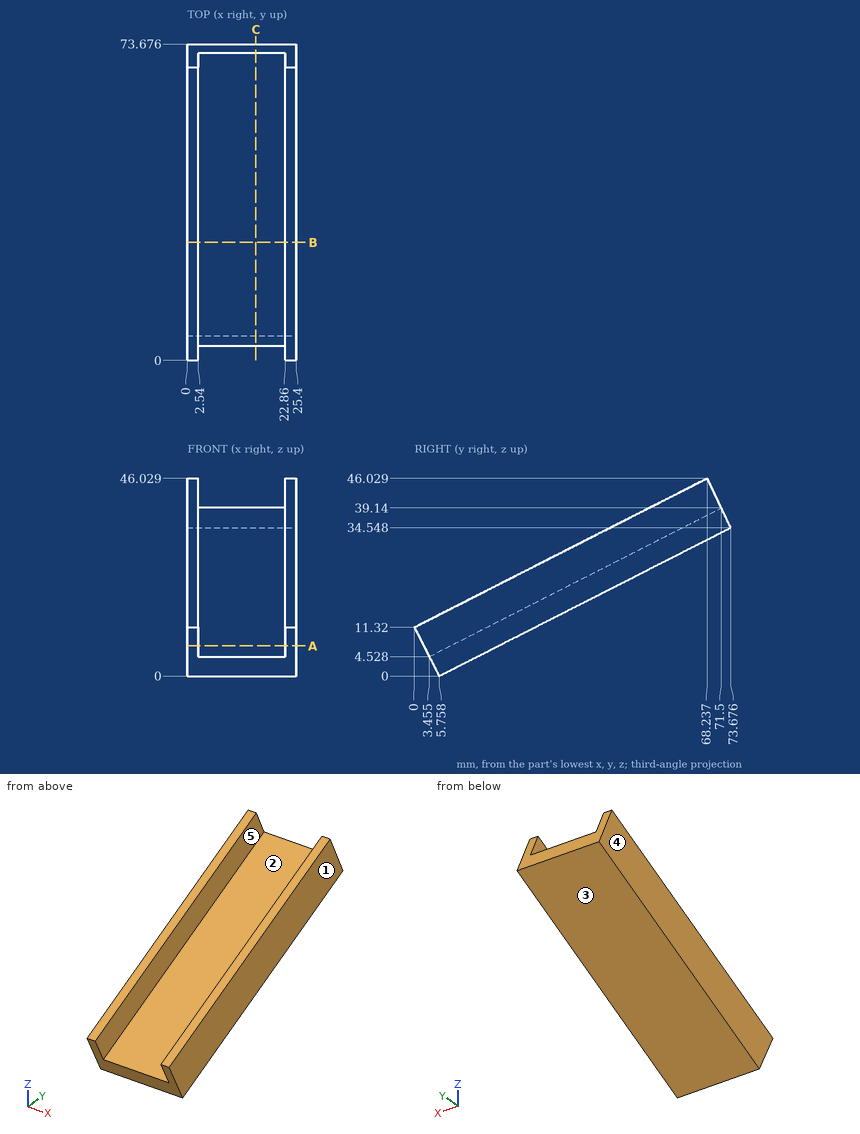
Study the drawing (mm; zero at the part's minimum x, y, z) and answer. A direction names the side the tool comes from. Round coordinates to 2 decimals unless told otherwise and drop trailing zeros. Write each loop counter-clockwise with the first axis right and the second up, starting at its lowest first coordinate (ties: lowest second). Pieces come first, ordered by that corner, then holes.
1) A cutting plane is placed at B-B (y = 27.5). Give the vertices of the cut face in (x, z), plus the area to 3 significant figures.
2) A cutting plane is placed at C-C (x = 16). Give the vertices of the cut face in (y, z) (1 decimal).
3) A cutting plane is placed at A-A (z = 7). Give the vertices of the cut face in (x, y) (1 decimal), plus the area to 3 significant figures.
4) Straight lines are drawn through the part: line 1 (Y direction, x = 2.75, z = 22) (1 decimal); line 2 (Y direction, x = 6, z = 2) (1 decimal); line 3 (Z direction, x = 3.5, y = 58) (1 decimal). For each, find the intervals that lie inside material, in ascending order.
5) Given pin 1 Ø1 at (x, z) = (11, 38) entering from -Y (1 decimal); pin 2 Ø10 at (x, z) = (14, 35) entering from -Y; pin 3 Ø8 at (x, y) = (17.5, 53) entering from +Z (1 decimal), each flat-ended and moving along its own axis, determine where each tip first touches the part or whether it passes through.
6) A tool of negligible diameter and unlimited length cuts with its end or side. For the marked faces 1 and 2, from which of +Z, -Z, +X, -X, +Y, -Y can it reach the whole face along a straight path? Write none if from no direction.
7) The mould has two halves that part along X. Classify the marked faces 3, 4 and 5: pulls with the +X half, pulls with the -X half, needs draft (parallel to the pull), parting line crosses it, or undercut.
Completed:
1. outline: (0, 11.06) - (25.4, 11.06) - (25.4, 25.31) - (22.86, 25.31) - (22.86, 16.76) - (2.54, 16.76) - (2.54, 25.31) - (0, 25.31) - close
1. area: 188 mm2
2. outline: (3.5, 4.5) - (5.8, 0) - (73.7, 34.5) - (71.5, 39.1) - close
3. outline: (0, 2.2) - (2.5, 2.2) - (2.5, 8.3) - (22.9, 8.3) - (22.9, 2.2) - (25.4, 2.2) - (25.4, 19.5) - (0, 19.5) - close
3. area: 316 mm2
4. line 1: y = 37.8 to 49
4. line 2: y = 4.7 to 9.7
4. line 3: z = 26.6 to 32.3
5. pin 1: stops at y = 68.3
5. pin 2: stops at y = 53.53
5. pin 3: stops at z = 31.8
6. face 1: +Z, -Z, +X, +Y, -Y
6. face 2: +Z, -Y
7. face 3: needs draft
7. face 4: pulls with the -X half
7. face 5: undercut
